Autodesk Inventor part; units mm, degrees
ref_plane "YZ Plane" through (0, 0, 0) normal (1, 0, 0) x (0, 1, 0)
ref_plane "XZ Plane" through (0, 0, 0) normal (0, 1, 0) x (-1, 0, 0)
ref_plane "XY Plane" through (0, 0, 0) normal (0, 0, 1) x (1, 0, 0)
sketch "Sketch1" plane through (0, 0, 0) normal (0, 1, 0) x (-1, 0, 0)
  line L0 (0, 0) -> (-8, 0)
  line L1 (-8, 0) -> (-8, -3.5)
  line L2 (-8, -3.5) -> (0, -3.5)
  line L3 (0, -3.5) -> (0, 0)
  dimension "d0" = 8
  dimension "d1" = 3.5
extrude "Extrusion1" add sketch "Sketch1" along normal blind 10
sketch "Sketch2" plane through (8, 0, -3.5) normal (0, 0, -1) x (-1, 0, 0)
  line L0 (0, 10) -> (8, 10)
  line L1 (3, 10) -> (5, 10)
  line L2 (5, 10) -> (5, 5)
  line L3 (5, 5) -> (3, 5)
  line L4 (3, 5) -> (3, 10)
  line L5 (8, 0) -> (8, 10)
  dimension "d4" = 2
  dimension "d5" = 5
  dimension "d6" = 3
extrude "Extrusion2" add sketch "Sketch2" along normal blind 3
sketch "Sketch3" plane through (5, 5, -3.5) normal (1, 0, 0) x (0, 0, -1)
  line L0 (0, 5) -> (3, 5)
  line L1 (0.8, 5) -> (3, 0.4)
  line L2 (3, 0) -> (3, 5)
  line L3 (0, -5) -> (0, 5)
  line L4 (0, 0) -> (3, 0)
  line L5 (0.8, 5) -> (3, 5)
  line L6 (3, 0.4) -> (3, 5)
  point P0 (-3.5, -5)
  dimension "d9" = 0.8
  dimension "d10" = 0.4
extrude "Extrusion3" cut sketch "Sketch3" against normal through all contours L0 L2 L1
properties part number "prueba"
The listing builds one solid part. Answer for the finished solid, in the listing's coordinates (mm). A direction names the side the tool comes from. Round coordinates to 2 decimals unless told otherwise and drop trailing zeros. Order: outer loops, then holes, each group sorted by start corner. A loop starts at its lowest first (then second) coordinate and runs counter-clockwise, first axis right, second up. Notation, with made-up numbers: (-40, 33.5) -> (2, 33.5) arc R17 ccw to (2, 55.5) -> close; hole circle Ø3 at (41.25, 11). An arc over 180 degrees is marked (long way). Answer as CSV lines item,"result". Start each with the question number.
(1) Flat-ended cylindrical pins translate along their axes: pin 1 Ø1.5 at (y, z) = (8.5, -4.5) entering from -X; pin 2 Ø0.9 at (y, z) = (6.5, -5) entering from +X; pin 3 Ø1.6 at (x, z) = (3.5, -5.5) entering from -Y. Find the tip coordinate at first contact, or state that the pin passes through.
(2) The part is cut by section C-C (y = 7.25). Determine the outline of the cut face in (x, z), then the cut area to 3 significant figures.
(3) The part is cut by section A-A (x = 4.25). Determine the outline of the cut face in (y, z), then the cut area to 3 significant figures.
(4) Find the intervals of material crossed by probe 1 along Z at (x, y) = (6.5, 2.25); probe 2 along X at (y, z) = (6.25, -5.5); probe 3 along Y at (x, z) = (3.75, -4.25), in increasing order. Write a range as from..to.
(5) A tool of negligible diameter and unlimited length cuts with its end or side. For faces 1 (the face through (3, 7, -5)), 2 (the face through (4, 10, -2)), 3 (the face through (4, 5, 0)), 4 (the face through (4, 5, -5)), 5 (the face through (5, 7, -5)), from which of +Z, -Z, +X, -X, +Y, -Y can it reach the whole face along a straight path? Write none if from no direction.
(6) The part is cut by section B-B (z = -4). Determine the outline of the cut face in (x, y), then the cut area to 3 significant figures.
(7) The part is cut by section D-D (x = 7). Determine the outline of the cut face in (y, z).
Evaluation:
1,pin 1,"x = 3"
1,pin 2,"x = 5"
1,pin 3,"y = 5"
2,outline,"(0, -3.5) -> (3, -3.5) -> (3, -5.62) -> (5, -5.62) -> (5, -3.5) -> (8, -3.5) -> (8, 0) -> (0, 0) -> close"
2,area,"32.2 mm²"
3,outline,"(0, -3.5) -> (5, -3.5) -> (5, -6.5) -> (5.4, -6.5) -> (10, -4.3) -> (10, 0) -> (0, 0) -> close"
3,area,"44.9 mm²"
4,probe 1,"-3.5..0"
4,probe 2,"3..5"
4,probe 3,"5..10"
5,face 1,"-Z, -X, +Y, -Y"
5,face 2,"+Z, -Z, +X, -X, +Y"
5,face 3,"+Z, +X, -X, +Y, -Y"
5,face 4,"-Z, +X, -X, -Y"
5,face 5,"-Z, +X, +Y, -Y"
6,outline,"(3, 5) -> (5, 5) -> (5, 10) -> (3, 10) -> close"
6,area,"10.0 mm²"
7,outline,"(0, -3.5) -> (10, -3.5) -> (10, 0) -> (0, 0) -> close"
